from build123d import *

# Parameters (mm, degrees)
SKETCH1_W           = 10
SKETCH1_H           = 20
SKETCH1_W_2         = 20
SKETCH1_H_2         = 10
BOSS_EXTRUDE1_DEPTH = 3


with BuildPart() as part:
    # Sketch1 → Boss-Extrude1 (new body)
    with BuildSketch(Plane(origin=(0, 0, 0), x_dir=(1, 0, 0), z_dir=(0, 1, 0))):
        Polygon((250, 100), (250, 150), (247, 150), (247, 200), (250, 200), (250, 250), (250, 253), (247, 253), (247, 250), (197, 250), (197, 253), (147, 253), (147, 250), (97, 250), (97, 253), (47, 253), (47, 250), (3, 250), (3, 253), (0, 253), (0, 250), (0, 200), (3, 200), (3, 150), (0, 150), (0, 100), (3, 100), (3, 50), (0, 50), (0, 0), (250, 0), (250, 50), (247, 50), (247, 100), align=None)
        with Locations((95, 150)):
            Rectangle(SKETCH1_W, SKETCH1_H, mode=Mode.SUBTRACT)
        with Locations((40, 150)):
            Rectangle(SKETCH1_W, SKETCH1_H, mode=Mode.SUBTRACT)
        with Locations((205, 95)):
            Rectangle(SKETCH1_W_2, SKETCH1_H_2, mode=Mode.SUBTRACT)
        with Locations((205, 40)):
            Rectangle(SKETCH1_W_2, SKETCH1_H_2, mode=Mode.SUBTRACT)
        with Locations((40, 205)):
            Rectangle(SKETCH1_W, SKETCH1_H, mode=Mode.SUBTRACT)
        with Locations((95, 205)):
            Rectangle(SKETCH1_W, SKETCH1_H, mode=Mode.SUBTRACT)
        with Locations((150, 95)):
            Rectangle(SKETCH1_W_2, SKETCH1_H_2, mode=Mode.SUBTRACT)
        with Locations((150, 40)):
            Rectangle(SKETCH1_W_2, SKETCH1_H_2, mode=Mode.SUBTRACT)
    extrude(amount=BOSS_EXTRUDE1_DEPTH)


solid = part.part
Design review of the part built by this model. Coordinates are the model's own, in mm. Round coordinates to 2 decimals unless told otherwise and drop trailing zeros. Order: outer loops, then holes, each group sorted by start corner. A loop starts at its lowest first (then second) coordinate and runs counter-clockwise, first axis right, second up. Notation, with made-up numbers: M 54.25,68.5 L 80.25,68.5 A20 cw 80.25,85.5 Z; hole C -21,46.25 d6. An arc over 180 degrees is marked long. Answer as CSV lines item,"result". Start each with the question number.
1) For pin 1 Ø1.5 at (x, y) = (94, 2) entering from +Z; pin 2 Ø1.5 at (y, z) = (1.5, -92.5) entering from -X; pin 3 Ø0.9 at (y, z) = (1, -185.5) entering from +X, all flat-tipped, find the tip position at first contact; note any pin that passes through.
2) Add section A-A (y = 1.55). Give the number of separate pieces and of enclosed holes in the cut face, then the cut area to 3 significant figures.
3) Wall thickness on line 1 along Z through (x, y) = (123, 2); line 2 along X through (y, z) = (1.9, -69.5): over which ranges is each line inside the solid? List them lowest first. Write a range as [from, to].
4) Add section B-B (z = -73.5). Give the boundary of the cut face in (x, y).
Resolved:
1,pin 1,"z = 0"
1,pin 2,"x = 3"
1,pin 3,"x = 247"
2,separate pieces,"1"
2,enclosed holes,"8"
2,area,"60,600 mm^2"
3,line 1,"[-250, 0]"
3,line 2,"[3, 247]"
4,outline,"M 3,0 L 247,0 L 247,3 L 3,3 Z"
